Read the model definition and answer for the solid it produces. Units are mm, in the model's axes. A direction names the side the tool comes from. Coordinates: 2 decimals unless noted, no trailing zeros. Loops run counter-clockwise (first coordinate to the right, second up) from the corner with the lowest first, then second, coordinate; pieces in that order, holes last. Notation, with made-up numbers: M 57,70 L 97,70 A22 cw 97,79 Z; hole C -15,60 d9. An arc over 180 degrees is marked long. Put each result on its own line as item: value.
from build123d import *

# Parameters (mm, degrees)
F0_W     = 77.094659
F0_H     = 92.319232
F1_DEPTH = 25.4
F2_R     = 16.165555
F3_DEPTH = 44.45
F5_DEPTH = 114.3


with BuildPart() as f1:
    # F0 (on Top) → F1 (new body)
    with BuildSketch(Plane.XY):
        with Locations((0.485893, 2.267493)):
            Rectangle(F0_W, F0_H)
    extrude(amount=F1_DEPTH)

    # F2 (on Top) → F3 (join)
    with BuildSketch(Plane.XY):
        Circle(F2_R)
    extrude(amount=F3_DEPTH)

    # F4 (on Front) → F5 (cut, symmetric)
    with BuildSketch(Plane.XZ):
        Polygon((39.681073, 63.003831), (-43.892127, 55.229578), (47.131397, 29.639332), align=None)
    extrude(amount=F5_DEPTH, both=True, mode=Mode.SUBTRACT)


solid = f1.part
1) Find section A-A, the plane y = 0. Write down the section's boundary in (x, z), plus the area to 3 significant figures.
Answer list:
outline: M -38.06,0 L 39.03,0 L 39.03,25.4 L 16.17,25.4 L 16.17,38.35 L -5.55,44.45 L -16.17,44.45 L -16.17,25.4 L -38.06,25.4 Z
area: 2,510 mm^2
2) Find section B-B, the plane x = -8. Write down the section's boundary in (y, z).
Answer list:
outline: M -43.89,0 L 48.43,0 L 48.43,25.4 L 14.05,25.4 L 14.05,44.45 L -14.05,44.45 L -14.05,25.4 L -43.89,25.4 Z
3) Straight lines are drawn through the part: line 1 (Z direction, x = 36, y = 30.5); line 2 (Y direction, x = 5, z = 39); line 3 (Y direction, x = 14.5, z = 31). For each, find the intervals that lie inside material, in ascending order. Write a range as [from, to].
Answer list:
line 1: z = [0, 25.4]
line 2: y = [-15.37, 15.37]
line 3: y = [-7.15, 7.15]
4) Given pin 1 Ø3 at (x, y) = (29.5, 32.5) entering from -Z; pin 2 Ø12 at (x, z) = (26.5, 36) entering from +Y; pin 3 Ø5 at (x, y) = (30, 2) entering from +Z, each flat-ended and moving along its own axis, determine where each tip first touches the part or whether it passes through.
Answer list:
pin 1: stops at z = 0
pin 2: passes through
pin 3: stops at z = 25.4
5) Find section D-D, the plane y = -24. Write down the section's boundary in (x, z), plus the area to 3 significant figures.
Answer list:
outline: M -38.06,0 L 39.03,0 L 39.03,25.4 L -38.06,25.4 Z
area: 1,960 mm^2
6) Which of the six approach directions +Z, -Z, +X, -X, +Y, -Y give full straight-line access (tool end or side, diameter ignored) to faces 1 (the flat face through (0, -43.892, 13)), 2 (the cylindrical face through (-16.15, 0.71, 34.79))?
Answer list:
face 1: +Z, -Z, +X, -X, -Y
face 2: +Z
7) Find section C-C, the plane x = 10. Write down the section's boundary in (y, z).
Answer list:
outline: M -43.89,0 L 48.43,0 L 48.43,25.4 L 12.7,25.4 L 12.7,40.08 L -12.7,40.08 L -12.7,25.4 L -43.89,25.4 Z
